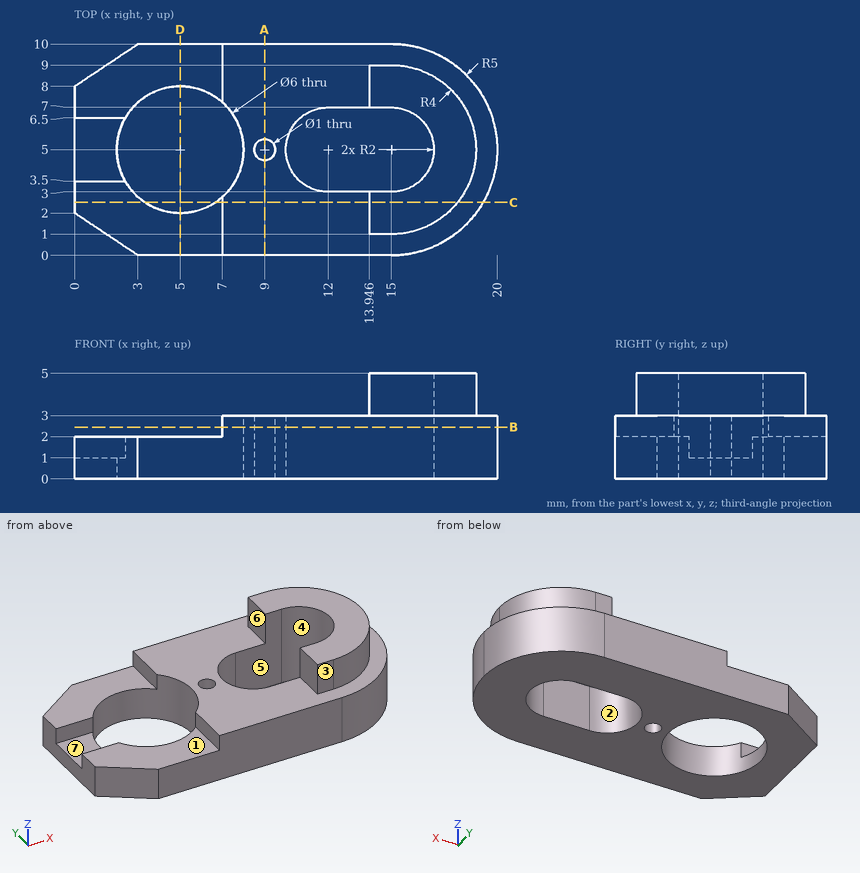
Here's the drawing with two shaded views (mm, measured from the low corner). I have some questions. A direction names the side the tool comes from. Coordinates: 2 decimals unless noted, no trailing zeros. Order: outer loops, then holes, each group sorted by start corner. A loop starts at its lowest first (then second) coordinate and runs counter-clockwise, first axis right, second up. Notation, with made-up numbers: (46.25, -2) - (64.25, -2) arc R18 ccw to (64.25, 18) - close; hole circle Ø5 at (5, -37). An arc over 180 degrees is marked (long way). Answer in a Markdown table with one row per item. Add a question column.
(1) If we section it at B-B, the plane z = 2.45: Please give me the cut outline in (x, y), then the cut area to 3 significant figures.
(2) Will these pins go through, and if not, where does the flat tip stop? pin 1 (1.2 mm diameter, centred on x = 14.5, z = 4, fed in from -Y); pin 2 (3 mm diameter, centred on x = 4.5, y = 9, fed in from +Z); pin 3 (0.5 mm diameter, centred on y = 2, z = 2.5, fed in from -X); pin 4 (1.5 mm diameter, centred on x = 13.5, z = 3.5, fed in from +Y).
(3) If we section it at C-C, the plane y = 2.5: Please give me the cut outline in (x, z).
(4) I need wall thicknesses on L1, parallel to Y at x = 9, z = 2.3; L2, parallel to Y at x = 5, z = 0.7; L3, parallel to Z at x = 9.25, y = 7.5. Which ranges of each line are inside material? Lowest first, please.
(5) On a 3-axis mill with a long thin cutter (end or side, diameter ignored), from which of +Z, -Z, +X, -X, +Y, -Y can I reach the whole of each face in a straight line? I mean the marked faces 1, 2 and 3. Say none if no direction works.
(6) If we section it at A-A, the plane x = 9: Please give me the cut outline in (y, z), then the cut area to 3 significant figures.
(7) If we mould it in two halves opening along X, with no side actions, what happens to the marked faces 4, 5, 6 and 7? For each: released by +X, released by -X, zero draft, split by the parting line, or undercut.
(8) If we section it at D-D, the plane x = 5: Please give me the cut outline in (y, z).
Results are:
| question | item | result |
|---|---|---|
| 1 | outline | (7, 0) - (15, 0) arc R5 ccw to (15, 10) - (7, 10) - (7, 7.24) arc R3 cw to (7, 2.76) - close; hole circle Ø1 at (9, 5); hole (12, 3) - (15, 3) arc R2 ccw to (15, 7) - (12, 7) arc R2 ccw to start |
| 1 | area | 90.8 mm2 |
| 2 | pin 1 | stops at y = 1 |
| 2 | pin 2 | stops at z = 2 |
| 2 | pin 3 | stops at x = 7 |
| 2 | pin 4 | stops at y = 10 |
| 3 | outline | (0, 0) - (3.34, 0) - (3.34, 2) - (0, 2) - close; (6.66, 0) - (19.33, 0) - (19.33, 3) - (18.12, 3) - (18.12, 5) - (13.95, 5) - (13.95, 3) - (7, 3) - (7, 2) - (6.66, 2) - close |
| 4 | L1 | y = 0 to 4.5, 5.5 to 10 |
| 4 | L2 | y = 0 to 2, 8 to 10 |
| 4 | L3 | z = 0 to 3 |
| 5 | face 1 | +Z, -X, +Y, -Y |
| 5 | face 2 | +Z, -Z |
| 5 | face 3 | +Z, +X, -X, -Y |
| 6 | outline | (0, 0) - (4.5, 0) - (4.5, 3) - (0, 3) - close; (5.5, 0) - (10, 0) - (10, 3) - (5.5, 3) - close |
| 6 | area | 27.0 mm2 |
| 7 | face 4 | undercut |
| 7 | face 5 | undercut |
| 7 | face 6 | released by -X |
| 7 | face 7 | zero draft |
| 8 | outline | (0, 0) - (2, 0) - (2, 2) - (0, 2) - close; (8, 0) - (10, 0) - (10, 2) - (8, 2) - close |
